from build123d import *

# Parameters (mm, degrees)
SKETCH_1_W          = 30
SKETCH_1_H          = 4
EXTRUDE_1_DEPTH     = 20
SKETCH_1_3_W        = 30
SKETCH_1_3_H        = 131
SKETCH_1_3_R        = 9.25
SKETCH_1_3_H_2      = 4
EXTRUDE_2_DEPTH     = 4
RIB_3_REACH         = 73.981
SKETCH_2_WALL_W     = 223.58267397
SKETCH_2_WALL_H     = 2
SKETCH_3_R          = 2.5
CUT_EXTRUDE_1_DEPTH = 4
FILLET_1_R          = 5
FILLET_2_R          = 2
FILLET_3_R          = 10


with BuildPart() as part:
    # Sketch 1 → Extrude 1 (new body)
    with BuildSketch(Plane.XY):
        with Locations((0, -65.5)):
            Rectangle(SKETCH_1_W, SKETCH_1_H)
    extrude(amount=EXTRUDE_1_DEPTH)

    # Sketch 1_3 → Extrude 2 (add)
    # profile 1 of 2: a face of its own
    with BuildSketch(Plane.XY):
        with Locations((0, 2)):
            Rectangle(SKETCH_1_3_W, SKETCH_1_3_H)
        with Locations((0, 52.5)):
            Circle(SKETCH_1_3_R, mode=Mode.SUBTRACT)
    # profile 2 of 2: a face of its own
    with BuildSketch(Plane.XY):
        with Locations((0, -65.5)):
            Rectangle(SKETCH_1_3_W, SKETCH_1_3_H_2)
    extrude(amount=-EXTRUDE_2_DEPTH)

    # Sketch 2 wall → Rib 3 (add, up to next)
    with BuildSketch(Plane(origin=(0, -26, 10), x_dir=(0, -0.966234939601, 0.25766265056), z_dir=(0, -0.25766265056, -0.966234939601)), mode=Mode.PRIVATE) as rib_3_sk1:
        Rectangle(SKETCH_2_WALL_W, SKETCH_2_WALL_H)
    rib_3_tool1 = extrude(rib_3_sk1.sketch, amount=RIB_3_REACH, mode=Mode.PRIVATE) - part.part
    add(rib_3_tool1.solids().sort_by_distance((0, -26, 10))[0])

    # Sketch 3 → Cut-Extrude 1 (cut)
    with BuildSketch(Plane.XZ.offset(67.5)):
        with Locations((-9, 10)):
            Circle(SKETCH_3_R)
        with Locations((9, 10)):
            Circle(SKETCH_3_R)
    extrude(amount=-CUT_EXTRUDE_1_DEPTH, mode=Mode.SUBTRACT)

    # Fillet 1
    fillet_1_edges = [part.edges().sort_by_distance(p)[0] for p in [
        (-15, -65.5, 20),
        (15, -65.5, 20),
    ]]
    fillet(fillet_1_edges, radius=FILLET_1_R)

    # Fillet 2
    fillet_2_edges = [part.edges().sort_by_distance(p)[0] for p in [
        (0, -67.5, -4),
        (8, -63.5, 0),
        (-8, -63.5, 0),
    ]]
    fillet(fillet_2_edges, radius=FILLET_2_R)

    # Fillet 3
    fillet_3_edges = [part.edges().sort_by_distance(p)[0] for p in [
        (-15, 67.5, -2),
        (15, 67.5, -2),
    ]]
    fillet(fillet_3_edges, radius=FILLET_3_R)


solid = part.part
For this review, take the finished solid that the model builds, in its own axes (mm). A direction names the side the tool comes from. Round coordinates to 2 decimals unless told otherwise and drop trailing zeros. Order: outer loops, then holes, each group sorted by start corner. A loop starts at its lowest first (then second) coordinate and runs counter-clockwise, first axis right, second up. Notation, with made-up numbers: (6, -17.75) -> (11, -17.75) arc R11 ccw to (11, -2.75) -> close; hole circle Ø4 at (-19, 24). An arc over 180 degrees is marked (long way). Write item = value, one per line. Start each with the question number.
1) The part is to be moulded in two halves that separate along Y. For faces 5 (the face through (-0.01, -25.47, 9.86)), 6 (the face through (-1, -36, 5)), 7 (the face through (0, -67.5, 9)), 8 (the face through (-1.2, 61.67, -1.97)), say which applies: +Y half, -Y half, draft (parallel to the pull), parting line (faces both ways), or undercut.
2) Tool access review of faces 1 (the face through (-6.5, -63.5, 10.9)), 2 (the face through (6, -63.5, 11)), 3 (the face through (-15, -15, -2)), 4 (the face through (-4, 4, 0)): name each direction out of +Z, -Z, +X, -X, +Y, -Y from which nothing blocks a thin tool from reaching the whole face with its end or side.
3) Take a section at A-A on y = 52.5. State the section outline as (x, z) points.
4) To check wall thickness, follow line 1 (Z direction, x = -9, y = -65.2); line 2 (Y direction, x = 0, z = -1.65); line 3 (Z direction, x = 7, y = 60.5). State the ranges of each line that lie inside material, in increasing order. Write a range as from..to.
5) Take a section at C-C on y = -38. State the section outline as (x, z) points, plus the area to 3 significant figures.
6) Take a section at B-B on z = 10. State the section outline as (x, y) points.
7) Insertion check: pin 1 (4 mm diameter, centred on x = -2.5, y = -35, fed in from +Z); pin 2 (4.5 mm diameter, centred on x = -9, z = 10, fed in from -Y). Each pin has a flat end and moves straight along its axis. Give the tip position at first contact, or say it passes through.
8) Take a section at D-D on z = 4.75. State the section outline as (x, y) points, plus the area to 3 significant figures.
Verdict:
q1.face_5 = +Y half
q1.face_6 = draft
q1.face_7 = -Y half
q1.face_8 = undercut
q2.face_1 = +Z, -X, +Y
q2.face_2 = +Z, +X, +Y
q2.face_3 = +Z, -Z, -X, +Y, -Y
q2.face_4 = +Z, +Y
q3.outline = (-15, -4) -> (-9.25, -4) -> (-9.25, 0) -> (-15, 0) -> close; (9.25, -4) -> (15, -4) -> (15, 0) -> (9.25, 0) -> close
q4.line_1 = -4..7.5, 12.5..20
q4.line_2 = -67.5..43.25, 61.75..67.5
q4.line_3 = -4..0
q5.outline = (-15, -4) -> (15, -4) -> (15, 0) -> (1, 0) -> (1, 13.2) -> (-1, 13.2) -> (-1, 0) -> (-15, 0) -> close
q5.area = 146 mm2
q6.outline = (-15, -67.5) -> (-11.5, -67.5) -> (-11.5, -63.5) -> (-15, -63.5) -> close; (-6.5, -67.5) -> (6.5, -67.5) -> (6.5, -63.5) -> (1, -63.5) -> (1, -26) -> (-1, -26) -> (-1, -63.5) -> (-6.5, -63.5) -> close; (11.5, -67.5) -> (15, -67.5) -> (15, -63.5) -> (11.5, -63.5) -> close
q7.pin_1 = 12.75
q7.pin_2 = through
q8.outline = (-15, -67.5) -> (15, -67.5) -> (15, -63.5) -> (1, -63.5) -> (1, -6.31) -> (-1, -6.31) -> (-1, -63.5) -> (-15, -63.5) -> close
q8.area = 234 mm2
